Design review of the part built by this model. Coordinates are the model's own, in mm. A direction names the side the tool comes from. Coordinates: 2 decimals unless noted, no trailing zeros. Write each loop counter-clockwise with the first axis right and the second up, starting at its lowest first coordinate (ties: lowest second). Pieces come first, ordered by that corner, then holes.
Q1. The part is to be moulded in two halves that separate along Y. For faces 1 (the flat face through (0, 0, -100)), 2 (the cylindrical face through (6.691, -12.864, 31.465)), 3 (the cylindrical face through (17.535, 13.24, -62.017)), 4 (the flat face through (15, 13, -64)), say which applies: released by +Y, released by -Y, zero draft, split by the parting line, or undercut.
Q2. Take a section at D-D, the plane z = 7.5. Write out the cut boundary in (x, y).
Q3. Take a section at B-B, the plane x = 17. Write out the cut boundary in (y, z).
Q4. For faces 5 (the flat face through (-18, -18, -5)), 6 (the flat face through (-16, 16, -2)), 7 (the cylindrical face through (17.535, -13.76, -62.017)), list the 3-axis set-ups (+Z, -Z, +X, -X, +Y, -Y) from which the entire face can be reached by the end or side of a thin tool; tool diameter is ignored.
Q5. For L1, parallel to Z at x = 18.05, y = -13.5; L2, parallel to Z at x = 18.8, y = -13.5; L3, parallel to Z at x = -7, y = -13, list the stretches that pass through material, from the lowest coordinate up.
Q6. Take a section at C-C, the plane x = 3. Write out the cut boundary in (y, z).
Q7. For pin 1 Ø2.5 at (x, y) = (-15, -15.5) entering from +Z; pin 2 Ø1.2 at (y, z) = (13, -11) entering from +X; pin 3 Ø6 at (x, z) = (-6.5, 4) entering from -Y, all flat-tipped, find the tip position at first contact; note any pin that passes through.
Q8. Take a section at A-A, the plane z = -10. Write out the cut boundary in (x, y).
from build123d import *

# Parameters (mm, degrees)
SKETCH_R        = 19
PAD_DEPTH       = 29
SKETCH001_W     = 40
SKETCH001_H     = 40
PAD001_DEPTH    = 100
POCKET_DEPTH    = 5
CHAMFER_SIZE    = 1
SKETCH003_R     = 14.5
PAD002_DEPTH    = 5
SKETCH016_R     = 15
PAD010_DEPTH    = 5
SKETCH014_R     = 2
POCKET001_DEPTH = 5


with BuildPart() as part:
    # Sketch → Pad (new body)
    with BuildSketch(Plane.XY):
        Circle(SKETCH_R)
    extrude(amount=PAD_DEPTH)

    # Sketch001 (on Face2 of Pad) → Pad001 (join)
    with BuildSketch(Plane(origin=(0, 0, 0), x_dir=(1, 0, 0), z_dir=(0, 0, -1))):
        Rectangle(SKETCH001_W, SKETCH001_H)
    extrude(amount=PAD001_DEPTH)

    # Sketch002 (on Face4 of Pad001) → Pocket (cut)
    with BuildSketch(Plane.XY):
        Polygon((-20, 12), (-20, 20), (-12, 20), align=None)
        Polygon((12, 20), (20, 20), (20, 12), align=None)
        Polygon((20, -12), (20, -20), (12, -20), align=None)
        Polygon((-12, -20), (-20, -20), (-20, -12), align=None)
    extrude(amount=-POCKET_DEPTH, mode=Mode.SUBTRACT)

    # Chamfer
    chamfer_edges = [part.edges().sort_by_distance(p)[0] for p in [
        (-20, -20, -52.5),
        (20, -20, -52.5),
        (20, 20, -52.5),
        (-20, 20, -52.5),
    ]]
    chamfer(chamfer_edges, length=CHAMFER_SIZE)

    # Sketch003 (on Face20 of Chamfer) → Pad002 (join)
    with BuildSketch(Plane.XY.offset(29)):
        Circle(SKETCH003_R)
    extrude(amount=PAD002_DEPTH)

    # Sketch016 (on Face22 of Pad002) → Pad010 (join)
    with BuildSketch(Plane.XY.offset(34)):
        Circle(SKETCH016_R)
    extrude(amount=PAD010_DEPTH)

    # Sketch014 (on Face11 of Chamfer) → Pocket001 (cut)
    with BuildSketch(Plane.YZ.offset(20)):
        with Locations((-13.5, -10)):
            Circle(SKETCH014_R)
        with Locations((13.5, -10)):
            Circle(SKETCH014_R)
        with Locations((13.5, -37)):
            Circle(SKETCH014_R)
        with Locations((-13.5, -37)):
            Circle(SKETCH014_R)
        with Locations((13.5, -64)):
            Circle(SKETCH014_R)
        with Locations((-13.5, -64)):
            Circle(SKETCH014_R)
    extrude(amount=-POCKET001_DEPTH, mode=Mode.SUBTRACT)


solid = part.part
Responses:
1. face 1: zero draft
1. face 2: split by the parting line
1. face 3: undercut
1. face 4: undercut
2. outline: circle Ø38 at (0, 0)
3. outline: (-20, -100) - (20, -100) - (20, -5) - (15, -5) - (15, 0) - (8.49, 0) - (8.49, 29) - (-8.49, 29) - (-8.49, 0) - (-15, 0) - (-15, -5) - (-20, -5) - close; hole circle Ø4 at (-13.5, -64); hole circle Ø4 at (-13.5, -37); hole circle Ø4 at (-13.5, -10); hole circle Ø4 at (13.5, -64); hole circle Ø4 at (13.5, -37); hole circle Ø4 at (13.5, -10)
4. face 5: +Z, -X, -Y
4. face 6: +Z, -X, +Y
4. face 7: +X
5. L1: z = -100 to -66, -62 to -39, -35 to -12, -8 to 0
5. L2: z = -100 to -66, -62 to -39, -35 to -12, -8 to -5
5. L3: z = -100 to 29, 34 to 39
6. outline: (-20, -100) - (20, -100) - (20, 0) - (18.76, 0) - (18.76, 29) - (14.19, 29) - (14.19, 34) - (14.7, 34) - (14.7, 39) - (-14.7, 39) - (-14.7, 34) - (-14.19, 34) - (-14.19, 29) - (-18.76, 29) - (-18.76, 0) - (-20, 0) - close
7. pin 1: stops at z = 0
7. pin 2: stops at x = 15
7. pin 3: stops at y = -18.67
8. outline: (-20, -19) - (-19, -20) - (19, -20) - (20, -19) - (20, -15.5) - (15, -15.5) - (15, -11.5) - (20, -11.5) - (20, 11.5) - (15, 11.5) - (15, 15.5) - (20, 15.5) - (20, 19) - (19, 20) - (-19, 20) - (-20, 19) - close
